```python
from build123d import *

# Parameters (mm, degrees)
F1_DEPTH = 15.24
F1_TAPER = 3.9
F3_DEPTH = 2.54
F4_R     = 3.3655
F5_DEPTH = 12.7
F6_R     = 4.6711310498
F6_R_2   = 3.429
F7_DEPTH = 12.7
F8_R     = 3.805331909
F9_DEPTH = 2.54
F10_SIZE = 0.762


with BuildPart() as f1:
    # F0 (on Top) → F1 (new body)
    with BuildSketch(Plane.XY):
        Polygon((-50.7999970374, 9.652), (-50.7999970374, 0), (3.175, 0), (3.175, 9.6704338458), align=None)
    extrude(amount=F1_DEPTH, taper=F1_TAPER)

    # F2 (on face) → F3 (join)
    with BuildSketch(Plane(origin=(0, 0, 0), x_dir=(1, 0, 0), z_dir=(0, 0, -1))):
        with BuildLine():
            ThreePointArc((-2.5432681699, -11.1761773853), (-1.1894436211, -11.3221739124), (0.1021277994, -11.7534501125))
            ThreePointArc((0.1021277994, -11.7534501125), (10.8966029626, -4.8261773853), (0.1021277994, 2.101095342))
            ThreePointArc((0.1021277994, 2.101095342), (-1.1894436211, 1.6698191419), (-2.5432681699, 1.5238226147))
            Line((-2.5432681699, 1.5238226147), (-52.0699970374, 1.5238226147))
            Line((-52.0699970374, 1.5238226147), (-52.0699970374, -11.1761773853))
            Line((-52.0699970374, -11.1761773853), (-2.5432681699, -11.1761773853))
        make_face()
    extrude(amount=-F3_DEPTH)

    # F4 (on face) → F5 (cut)
    with BuildSketch(Plane(origin=(0, 0, 0), x_dir=(1, 0, 0), z_dir=(0, 0, -1))):
        with Locations((3.2766029626, -4.8261773853)):
            Circle(F4_R)
    extrude(amount=-F5_DEPTH, mode=Mode.SUBTRACT)

    # F6 (on face) → F7 (join)
    with BuildSketch(Plane.XY.offset(2.54)):
        with Locations((3.2766029626, 4.8261773853)):
            Circle(F6_R)
        with Locations((3.2766029626, 4.8261773853)):
            Circle(F6_R_2, mode=Mode.SUBTRACT)
    extrude(amount=F7_DEPTH)

    # F8 (on face) → F9 (join)
    with BuildSketch(Plane.XY.offset(15.24)):
        with Locations((3.2766029626, 4.8261773853)):
            Circle(F8_R)
    extrude(amount=-F9_DEPTH)

    # F10
    f10_edges = [f1.edges().sort_by_distance(p)[0] for p in [
        (-1.189444, 11.322174, 0),
        (-27.306633, 11.176177, 0),
        (10.896603, 4.826177, 0),
        (-52.069997, 4.826177, 0),
        (-1.189444, -1.669819, 0),
        (-27.306633, -1.523823, 0),
        (-0.088897, 4.826177, 0),
    ]]
    chamfer(f10_edges, length=F10_SIZE)


solid = f1.part
```
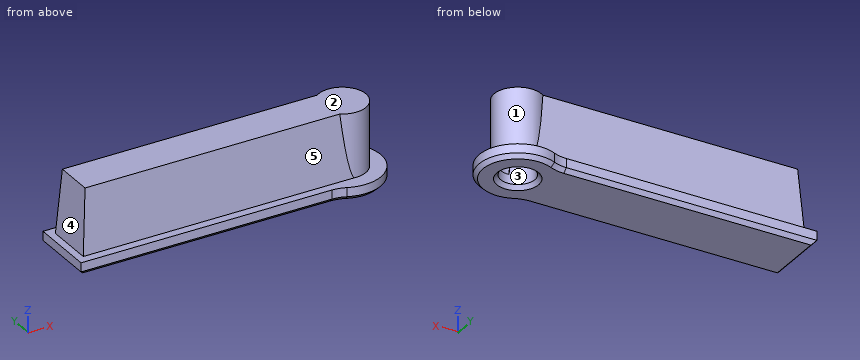
Here's how the part is built. I have some questions about the finished solid (model axes, mm). Face numbers are marked on the shaded views. A direction names the side the tool comes from. Give positions to 0.01 mm unless a question says otherwise; leave off trailing zeros. Order: outer loops, then holes, each group sorted by start corner. A loop starts at its lowest first (then second) coordinate and runs counter-clockwise, first axis right, second up. Notation, with made-up numbers: M 59.5,4.5 L 101.5,4.5 A29 ccw 101.5,24.5 Z; hole C 0,4 d4. An arc over 180 degrees is marked long. Use a Markdown table: item, result. Add a question column.
1. Suppose I cut it at B-B (x = -19). List the corners of the cut face in (y, z) for me, and give its area (3 significant figures).
2. For pin 1 Ø2 at (x, z) = (-23.5, 1.5) entering from -Y; pin 2 Ø2 at (x, z) = (-31.5, 11) entering from -Y; pin 3 Ø4 at (x, z) = (-33, 2) entering from +Y, each with a flat end and sliding along its axis, tell me the tip position at first contact or that it passes through.
3. Suppose I cut it at C-C (z = 6). List the corners of the cut face in (x, y) for me.
4. Suppose I cut it at A-A (z = 9). List the corners of the cut face in (x, y) for me, and give its area (3 significant figures).
5. On a 3-axis mill with a long thin cutter (end or side, diameter ignored), from which of +Z, -Z, +X, -X, +Y, -Y can I reach the whole of each face in a straight line? I mean the marked faces 1 and 2. Say none if no direction works.
6. I need wall thicknesses on probe 1 along Z at (x, y) = (-48.5, 10.25); probe 2 along Y at (x, z) = (-31.5, 1.25); probe 3 along X at (y, z) = (6.75, 6.5). Which ranges of each line are inside material? Lowest first, please. Write a range as from..to.
7. If we mould it in two halves opening along X, with no side actions, what happens to the marked faces 3, 4 and 5? For each: +X half, -X half, draft (parallel to the pull), parting line (faces both ways), or undercut.
8. Suppose I cut it at D-D (x = -11). List the corners of the cut face in (y, z) for me.
Results list:
| question | item | result |
|---|---|---|
| 1 | outline | M -1.52,0.76 L -0.76,0 L 10.41,0 L 11.18,0.76 L 11.18,2.54 L 9.49,2.54 L 8.62,15.24 L 1.04,15.24 L 0.17,2.54 L -1.52,2.54 Z |
| 1 | area | 139 mm² |
| 2 | pin 1 | stops at y = -1.52 |
| 2 | pin 2 | stops at y = 0.68 |
| 2 | pin 3 | stops at y = 11.18 |
| 3 | outline | M -50.39,0.41 L 1.76,0.41 A4.67 ccw long 1.81,9.26 L -50.39,9.24 Z; hole M 2.77,1.44 A3.43 ccw long 2.77,8.22 L 2.77,8.15 A3.37 ccw 2.77,1.5 Z |
| 4 | outline | M -50.19,0.61 L 1.26,0.61 A4.67 ccw long 1.3,9.06 L -50.19,9.04 Z; hole M 2.56,1.47 A3.43 ccw long 2.56,8.18 L 2.56,8.11 A3.37 ccw 2.56,1.54 Z |
| 4 | area | 450 mm² |
| 5 | face 1 | +Z |
| 5 | face 2 | +Z, +X, -X, +Y, -Y |
| 6 | probe 1 | z = 0..2.54 |
| 6 | probe 2 | y = -1.52..11.18 |
| 6 | probe 3 | x = -50.36..0.52, 6.12..7.53 |
| 7 | face 3 | undercut |
| 7 | face 4 | -X half |
| 7 | face 5 | draft |
| 8 | outline | M -1.52,0.76 L -0.76,0 L 10.41,0 L 11.18,0.76 L 11.18,2.54 L 9.49,2.54 L 8.63,15.24 L 1.04,15.24 L 0.17,2.54 L -1.52,2.54 Z |
